from build123d import *

# Parameters (mm, degrees)
CROQUIS1_R                 = 7.95
SALIENTE_EXTRUIR1_DEPTH    = 7.5
CROQUIS2_R                 = 8.45
SALIENTE_EXTRUIR2_DEPTH    = 0.5
SALIENTE_EXTRUIR3_START    = -14.5
CROQUIS2_2_R               = 8.45
SALIENTE_EXTRUIR3_DEPTH    = 0.5
CROQUIS3_R                 = 5
SALIENTE_EXTRUIR4_DEPTH    = 21
CORTAR_EXTRUIR1_DEPTH      = 24.728779994
CORTAR_EXTRUIR1_DEPTH_BACK = 24.728779994
CROQUIS4_R                 = 3
CROQUIS7_W                 = 1.25
CROQUIS7_H                 = 5
CROQUIS9_W                 = 1.25
CROQUIS9_H                 = 8.45


with BuildPart() as part:
    # Croquis1 → Saliente-Extruir1 (new, symmetric)
    with BuildSketch(Plane(origin=(0, 0, 0), x_dir=(-1, 0, 0), z_dir=(0, 1, 0))):
        with Locations(Location((0, 0, 0), (0, 0, 90))):
            Circle(CROQUIS1_R)
    extrude(amount=SALIENTE_EXTRUIR1_DEPTH, both=True)

    # Croquis2 → Saliente-Extruir2 (add)
    with BuildSketch(Plane(origin=(0, 7.5, 0), x_dir=(-1, 0, 0), z_dir=(0, 1, 0))):
        with Locations(Location((0, 0, 0), (0, 0, 90))):
            Circle(CROQUIS2_R)
    extrude(amount=-SALIENTE_EXTRUIR2_DEPTH)

    # Croquis2<2> → Saliente-Extruir3 (add)
    with BuildSketch(Plane(origin=(0, 7.5, 0), x_dir=(-1, 0, 0), z_dir=(0, 1, 0)).offset(SALIENTE_EXTRUIR3_START)):
        with Locations(Location((0, 0, 0), (0, 0, 90))):
            Circle(CROQUIS2_2_R)
    extrude(amount=-SALIENTE_EXTRUIR3_DEPTH)

    # Croquis3 → Saliente-Extruir4 (add)
    with BuildSketch(Plane(origin=(0, -7.5, 0), x_dir=(-1, 0, 0), z_dir=(0, 1, 0))):
        with Locations(Location((0, 0, 0), (0, 0, 270))):
            Circle(CROQUIS3_R)
    extrude(amount=SALIENTE_EXTRUIR4_DEPTH)

    # Croquis4 → Cortar-Extruir1 (cut, two sides: drawn at the far end of the back side and taken through both)
    with BuildSketch(Plane(origin=(0, -7, 0), x_dir=(-1, 0, 0), z_dir=(0, 1, 0)).offset(-CORTAR_EXTRUIR1_DEPTH_BACK)):
        with Locations(Location((0, 0, 0), (0, 0, 90))):
            Circle(CROQUIS4_R)
    extrude(amount=CORTAR_EXTRUIR1_DEPTH + CORTAR_EXTRUIR1_DEPTH_BACK, mode=Mode.SUBTRACT)

    # Croquis7 → Taladro roscado M32 (revolve, cut)
    with BuildSketch(Plane.ZX.offset(10.5)):
        with Locations((0.625, 2.5)):
            Rectangle(CROQUIS7_W, CROQUIS7_H)
    revolve(axis=Axis((-6.35, 10.5, 0), (1, 0, 0)), mode=Mode.SUBTRACT)

    # Croquis9 → Taladro roscado M31 (revolve, cut)
    with BuildSketch(Plane(origin=(0, 10.5, 0), x_dir=(0, 1, 0), z_dir=(1, 0, 0))):
        with Locations((0.625, 4.225)):
            Rectangle(CROQUIS9_W, CROQUIS9_H)
    revolve(axis=Axis((0, 10.5, -6.35), (0, 0, 1)), mode=Mode.SUBTRACT)


solid = part.part
Can you work these out from the model? Positions are in its coordinate system, mm. A direction names the side the tool comes from. Give positions to 0.01 mm unless a question says otherwise; leave off trailing zeros. Order: outer loops, then holes, each group sorted by start corner. A loop starts at its lowest first (then second) coordinate and runs counter-clockwise, first axis right, second up. Notation, with made-up numbers: M 29.25,63 L 43.25,63 A9 ccw 43.25,74 Z; hole C 69.5,19 d5. An arc over 180 degrees is marked long. Use a Markdown table: item, result. Add a question column.
Item 1: If I drill on L1, parallel to Y at x = 4.25, z = 0; L2, parallel to Y at x = 6.75, z = -3; L3, parallel to Y at x = 1, z = 3.5, over which ranges is the centre line in solid material (lowest first)? Write a range as [from, to].
Item 2: Suppose I cut it at C-C (y = 10). List the corners of the cut face in (x, z) for me.
Item 3: Suppose I cut it at B-B (z = 0). List the corners of the cut face in (x, y) for me, then the cut area to 4 significant figures.
Item 4: Suppose I cut it at A-A (x = 0). List the corners of the cut face in (y, z) for me.
Item 5: We'd pull the mould along Y, two halves only. Please class faces 1 (the cylindrical face through (3.88, 10.45, -1.25)), 2 (the flat face through (3.3, 13.5, 0.1)), 3 (the cylindrical face through (2.54, -7.25, 8.06)): +Y half, -Y half, draft (parallel to the pull), parting line (faces both ways), or undercut.
Item 6: Will these pins go through, and if not, where does the flat tip stop? pin 1 (1 mm diameter, centred on x = -5.5, z = 1, fed in from +Y); pin 2 (1.5 mm diameter, centred on y = 3, z = 1.5, fed in from +X); pin 3 (1.5 mm diameter, centred on y = 10.5, z = 0, fed in from +X); pin 4 (5 mm diameter, centred on x = 0, z = 0, fed in from -Y).
Item 7: Suppose I cut it at D-D (y = 1.5). List the corners of the cut face in (x, z) for me, then the cut area to 3 significant figures.
Item 8: For faces 4 (the flat face through (0, -7.5, -4)), 5 (the cylindrical face through (-4.837, 0.098, -6.309)), 6 (the cylindrical face through (-0.05, 9.25, 3.88)), 7 (the cylindrical face through (-1.5, 10.46, -4.77)), which set-ups out of +Z, -Z, +X, -X, +Y, -Y let a thin tool reach every point of the face, with its end or its side?
Answer sheet:
| question | item | result |
|---|---|---|
| 1 | L1 | y = [-7.5, 9.25], [11.75, 13.5] |
| 1 | L2 | y = [-7.5, 7.5] |
| 1 | L3 | y = [-7.5, 9.75], [11.25, 13.5] |
| 2 | outline | M -1.15,2.77 L -1.15,4.87 A5 ccw long 4.87,-1.15 L 2.77,-1.15 A3 cw long Z; M 1.15,2.77 A3 cw 2.77,1.15 L 4.87,1.15 A5 ccw 1.15,4.87 Z |
| 3 | outline | M -8.45,-7.5 L -3,-7.5 L -3,13.5 L -5,13.5 L -5,7.5 L -8.45,7.5 L -8.45,7 L -7.95,7 L -7.95,-7 L -8.45,-7 Z; M 3,-7.5 L 8.45,-7.5 L 8.45,-7 L 7.95,-7 L 7.95,7 L 8.45,7 L 8.45,7.5 L 5,7.5 L 5,9.25 L 3,9.25 Z; M 3,11.75 L 5,11.75 L 5,13.5 L 3,13.5 Z |
| 3 | area | 168.5 mm² |
| 4 | outline | M -7.5,-8.45 L -7,-8.45 L -7,-7.95 L 7,-7.95 L 7,-8.45 L 7.5,-8.45 L 7.5,-5 L 13.5,-5 L 13.5,-3 L -7.5,-3 Z; M -7.5,3 L 9.25,3 L 9.25,5 L 7.5,5 L 7.5,8.45 L 7,8.45 L 7,7.95 L -7,7.95 L -7,8.45 L -7.5,8.45 Z; M 11.75,3 L 13.5,3 L 13.5,5 L 11.75,5 Z |
| 5 | face 1 | undercut |
| 5 | face 2 | +Y half |
| 5 | face 3 | draft |
| 6 | pin 1 | stops at y = 7.5 |
| 6 | pin 2 | stops at x = 7.91 |
| 6 | pin 3 | stops at x = -2.9 |
| 6 | pin 4 | passes through |
| 7 | outline | C 0,0 d15.9; hole C 0,0 d6 |
| 7 | area | 170 mm² |
| 8 | face 4 | +Z, -Z, +X, -X, -Y |
| 8 | face 5 | none |
| 8 | face 6 | +Z |
| 8 | face 7 | +Y |
